Autodesk Inventor part; units mm, degrees
ref_plane "YZ Plane" through (0, 0, 0) normal (1, 0, 0) x (0, 1, 0)
ref_plane "XZ Plane" through (0, 0, 0) normal (0, 1, 0) x (-1, 0, 0)
ref_plane "XY Plane" through (0, 0, 0) normal (0, 0, 1) x (1, 0, 0)
sketch "Sketch1" plane through (0, 0, 0) normal (0, 0, 1) x (1, 0, 0)
  line L0 (-19.2849, 35) -> (-19.2849, -35) construction
  line L1 (19.7114, 54.5) -> (19.7114, -54.5) construction
  line L2 (-19.2849, 35) -> (19.7114, 54.5) construction
  line L3 (-19.2849, -35) -> (19.7114, -54.5) construction
  circle A0 centre (0.08, 0) radius 14.5
  line L4 (-19.2849, 35) -> (0.08, 0) construction
  line L5 (0.08, 0) -> (-19.2849, -35) construction
  circle A1 centre (19.7114, 54.5) radius 1.6 construction
  circle A2 centre (-19.2849, 35) radius 1.6 construction
  circle A3 centre (-19.2849, -35) radius 1.6 construction
  circle A4 centre (19.7114, -54.5) radius 1.6 construction
  line L6 (-16, -69) -> (0, -69)
  line L7 (0, 69) -> (-16, 69)
  arc A5 (-16, 69) -> (-16, -69) centre (-16, 0) ccw
  arc A6 (0, -69) -> (0, 69) centre (0, 0) ccw
  line L8 (-85, 0) -> (69, 0) construction
  circle A7 centre (-19.2849, 35) radius 3 construction
  circle A8 centre (-19.2849, -35) radius 3 construction
  circle A9 centre (19.7114, 54.5) radius 3 construction
  circle A10 centre (19.7114, -54.5) radius 3 construction
  line L9 (0.08, 60) -> (0.08, -60) construction
  line L10 (-55, -40) -> (-55, 40) construction
  circle A11 centre (-55, 40) radius 2.25
  circle A12 centre (-55, -40) radius 2.25
  circle A13 centre (0.08, -60) radius 2.25
  circle A14 centre (0.08, 60) radius 2.25
  point P0 (-19.2849, 0)
  point P1 (19.7114, 0)
  point P2 (-55, 0)
  dimension "d0" = 70
  dimension "d1" = 109
  dimension "d2" = 43.6
  dimension "d3" = 29
  dimension "d4" = 40
  dimension "d5" = 3.2
  dimension "d7" = 138
  dimension "d8" = 154
  dimension "d33" = 6
  dimension "d55" = 85.08
  dimension "d74" = 80
  dimension "d76" = 30
  dimension "d77" = 4.5
  dimension "d78" = 120
extrude "Extrusion1" add sketch "Sketch1" along normal blind 11 contours A5 L7 A6 L6 | A11 | A12 | A13 | A14
sketch "Sketch2" plane through (0, 0, 11) normal (0, 0, 1) x (1, 0, 0)
  circle A0 centre (-52.47, 0) radius 18.5329 construction
  circle A1 centre (-71.0029, 0) radius 1.25
  circle A2 centre (-43.2035, 16.05) radius 1.25
  circle A3 centre (-43.2035, -16.05) radius 1.25
  circle A4 centre (0.08, 0) radius 14.5
  line L0 (-16, -69) -> (0, -69)
  arc A5 (0, -69) -> (0, 69) centre (0, 0) ccw
  line L1 (0, 69) -> (-16, 69)
  arc A6 (-16, 69) -> (-16, -69) centre (-16, 0) ccw
  arc A7 (-16, 69) -> (-16, -69) centre (-16, 0) ccw construction
  line L2 (-85, 0) -> (69, 0) construction
  circle A8 centre (-43.2035, -16.05) radius 5
  circle A9 centre (-43.2035, 16.05) radius 5
  circle A10 centre (-71.0029, 0) radius 5
  circle A11 centre (-52.47, 0) radius 16.25
  line L3 (-53.47, -16.2192) -> (-53.47, -23.7192)
  line L4 (-53.47, -23.7192) -> (-51.47, -23.7192)
  line L5 (-51.47, -23.7192) -> (-51.47, -16.2192)
  line L6 (-52.47, -23.7192) -> (-52.47, 0) construction
  arc A12 (-53.47, -16.2192) -> (-51.47, -16.2192) centre (-52.47, 0) ccw
  dimension "d67" = 32.5
  dimension "d11" = 120
  dimension "d12" = 120
  dimension "d13" = 32.1
  dimension "d14" = 52.55
  dimension "d40" = 2.5
  dimension "d49" = 10
  dimension "d97" = 7.5
  dimension "d98" = 2
sketch "Sketch3" plane through (0, 0, 0) normal (0, 0, -1) x (-1, 0, 0)
  circle A0 centre (30.8533, 41.3) radius 6
  circle A1 centre (-0.08, 0) radius 14.5
  circle A2 centre (30.8533, -41.3) radius 6
  line L0 (30.8533, 41.3) -> (-0.08, 0) construction
  line L1 (-0.08, 0) -> (30.8533, -41.3) construction
  circle A3 centre (-38.88, 0) radius 55.5
  circle A4 centre (-0.08, 0) radius 14.5 construction
  line L2 (16, -69) -> (0, -69) construction
  arc A5 (16, -69) -> (16, 69) centre (16, 0) ccw construction
  line L3 (0, 69) -> (16, 69) construction
  arc A6 (0, 69) -> (0, -69) centre (0, 0) ccw construction
  arc A7 (16, -69) -> (16, 69) centre (16, 0) ccw construction
  line L4 (85, 0) -> (-129.38, 0) construction
  arc A8 (0, 69) -> (0, -69) centre (0, 0) ccw construction
  line L5 (30.8533, 41.3) -> (30.8533, -41.3)
  line L6 (37.1783, 47.625) -> (-131.38, 47.625)
  line L7 (-131.38, 47.625) -> (-131.38, -47.625)
  line L8 (-131.38, -47.625) -> (37.1783, -47.625)
  line L9 (37.1783, -47.625) -> (37.1783, 47.625)
  line L10 (30.8533, 41.3) -> (37.1783, 41.3) construction
  line L11 (30.8533, 41.3) -> (30.8533, 47.625) construction
  line L12 (30.8533, -41.3) -> (37.1783, -41.3) construction
  line L13 (30.8533, -41.3) -> (30.8533, -47.625) construction
  circle A9 centre (-107.4467, 41.3) radius 6
  circle A10 centre (-107.4467, -41.3) radius 6
  line L14 (30.8533, 41.3) -> (-107.4467, 41.3) construction
  line L15 (30.8533, -41.3) -> (-107.4467, -41.3) construction
  circle A11 centre (-111.88, 0) radius 17.5
  line L16 (-111.88, 17.5) -> (-91.5488, 17.5)
  line L17 (-111.88, -17.5) -> (-91.5488, -17.5)
  circle A12 centre (-38.88, 0) radius 57.5
  line L18 (-131.38, 0) -> (-129.38, 0)
  line L19 (-111.88, 17.5) -> (-111.88, -17.5) construction
  line L20 (-113.4467, 41.3) -> (-113.4467, 47.625)
  line L21 (-101.4467, 41.3) -> (-101.4467, 47.625)
  line L22 (-113.4467, 41.3) -> (-101.4467, 41.3)
  line L23 (-113.4467, 47.625) -> (-101.4467, 47.625)
  line L24 (-113.4467, -41.3) -> (-113.4467, -47.625)
  line L25 (-113.4467, -47.625) -> (-101.4467, -47.625)
  line L26 (-101.4467, -47.625) -> (-101.4467, -41.3)
  line L27 (-101.4467, -41.3) -> (-113.4467, -41.3)
  dimension "d15" = 51.6
  dimension "d17" = 111
  dimension "d18" = 82.6
  dimension "d22" = 95.25
  dimension "d29" = 138.3
  dimension "d30" = 35
  dimension "d59" = 2
  dimension "d60" = 12
  dimension "d81" = 2
  dimension "d99" = 38.8
extrude "Extrusion4" add sketch "Sketch3" against normal up to surface (11 mm away)
extrude "Extrusion14" cut sketch "Sketch3" against normal blind 6 contours A0 | A2 | L22 A9 | A9 L22 | L27 A10 | A10 L27
extrude "Extrusion15" cut sketch "Sketch3" against normal blind 10 contours A3 L6 L8 | A3 A11 A12 L16 | A11 A12 | A3 L17 A12 A11 | A3 L6 | A12 A11 L16 | A12 A11 | A12 L17 A11 | L8 A3
extrude "Extrusion16" cut sketch "Sketch2" against normal through all contours A1 | A2 | A3
extrude "Extrusion17" cut sketch "Sketch2" against normal blind 3 contours A11 A8 | A8 A11 A10 A9 | L5 L4 L3 A11 | A9 A11 | A11 A10 picked at (-44.8177, -13.2541) picked at (-44.8177, 13.2541) picked at (-67.7746, 0)
fillet "Fillet1" radius 5 1 edges at (131.38, -47.625, 5.5)
fillet "Fillet2" radius 5 1 edges at (131.38, 47.625, 5.5)
extrude "Extrusion20" cut sketch "Sketch1" along normal through all contours A11 | A12 | A13 | A14
sketch "Sketch10" plane through (0, 0, 11) normal (0, 0, 1) x (1, 0, 0)
  circle A0 centre (0.08, -60) radius 2.25
  circle A1 centre (0.08, 60) radius 2.25
  circle A2 centre (-55, 40) radius 2.25
  circle A3 centre (-55, -40) radius 4
  circle A4 centre (0.08, -60) radius 4
  circle A5 centre (0.08, 60) radius 2.25
  circle A6 centre (0.08, 60) radius 4
  circle A7 centre (-55, 40) radius 4
  point P0 (0, 0)
  dimension "d88" = 8
extrude "Extrusion21" cut sketch "Sketch10" against normal blind 5
thread "Thread1"
thread "Thread2"
thread "Thread3"
extrude "Extrusion22" cut sketch "Sketch3" against normal up to surface (6 mm away) contours L21 A9 L20 L6 | L8 L24 A10 L26
properties part number "AZ-FLDIC-FWup bottom adapter"
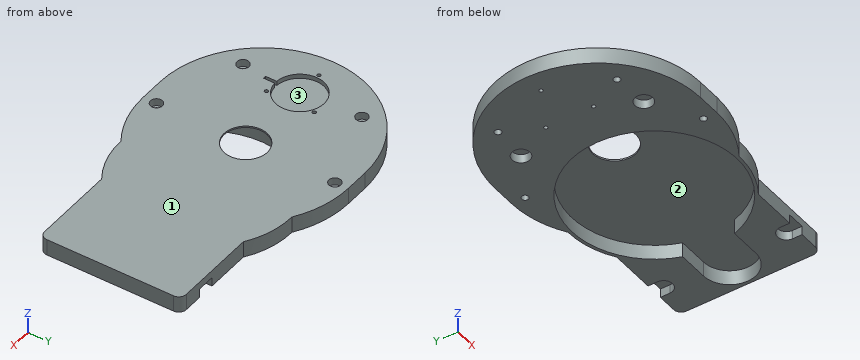
Work out the finished part from the listing and answer in its coordinate system (mm). Face numbers are marked on the shaded views. Coordinates: 2 decimals unless noted, no trailing zeros. Order: outer loops, then holes, each group sorted by start corner. A loop starts at its lowest first (then second) coordinate and runs counter-clockwise, first axis right, second up. Notation, with made-up numbers: (60.25, 2.5) - (104.25, 2.5) arc R8 ccw to (104.25, 17.5) - close; hole circle Ø9 at (19, -9). An arc over 180 degrees is marked (long way). Put each result on its own line as item: value. Start each with the question number.
1) Find section A-A (y = 60). Give the vertices of the cut face in (x, z).
2) Flat-ended cylindrical pins translate along their axes: pin 1 (5 mm diameter, centred on x = 102.5, z = 7, fed in from -Y) (3 decimals); pin 2 (2.5 mm diameter, centred on x = 0.08, y = 60, fed in from -Z); pin 3 (6 mm diameter, centred on x = -55, y = 40, fed in from +Z); pin 4 (3 mm diameter, centred on y = -43, z = 3, fed in from -X). Find the tip coordinate at first contact, or state that the pin passes through.
3) Find section C-C (x = 75). Give the vertices of the cut face in (y, z) (3 decimals).
4) For a pull along X with two mould halves and no side action, classify the marked faces 1, 2 and 3 as released by +X, released by -X, zero draft, split by the parting line, or undercut.
5) Find section D-D (y = 23.5). Give the vertices of the cut face in (x, z), plus the area to 3 significant figures.
6) Find the intervals of material crossed by line 1 (Y direction, x = -26, z = 2.25); line 2 (Y direction, x = -56.5, z = 0.5); line 3 (X direction, y = -11, z = 8.5), in increasing order. Write a range as from..to.
7) Find section B-B (z = 3). State how many separate pieces and enclosed holes the cut face has, plus the area to 3 significant figures.
Results list:
1. outline: (-50.07, 0) - (-2.17, 0) - (-2.17, 6) - (-3.92, 6) - (-3.92, 11) - (-50.07, 11) - close; (2.33, 0) - (34.07, 0) - (34.07, 11) - (4.08, 11) - (4.08, 6) - (2.33, 6) - close
2. pin 1: stops at y = -47.625
2. pin 2: passes through
2. pin 3: stops at z = 6
2. pin 4: stops at x = -71.12
3. outline: (-47.625, 0) - (-42.138, 0) - (-42.138, 10) - (42.138, 10) - (42.138, 0) - (47.625, 0) - (47.625, 11) - (-47.625, 11) - close
4. face 1: zero draft
4. face 2: undercut
4. face 3: undercut
5. outline: (-80.87, 0) - (-11.4, 0) - (-11.4, 10) - (89.16, 10) - (89.16, 0) - (131.38, 0) - (131.38, 11) - (-80.87, 11) - close
5. area: 1,330 mm^2
6. line 1: y = -68.27..-44.83, -37.77..37.77, 44.83..68.27
6. line 2: y = -55.86..-41.68, -38.32..38.32, 41.68..55.86
6. line 3: x = -84.12..-64.43, -40.51..-15.52, 125.49..131.38
7. separate pieces: 1
7. enclosed holes: 10
7. area: 12,600 mm^2
